Work out the finished part from the listing and answer in its coordinate system (mm). A direction names the side the tool comes from. Give positions to 0.01 mm unless a question says otherwise; leave off trailing zeros. Loops run counter-clockwise (first coordinate to the right, second up) from the corner with the lowest first, then second, coordinate; pieces in that order, holes last. Notation, with made-up numbers: (50, 39.25) - (85, 39.25) arc R18 ccw to (85, 66.25) - close; hole circle Ø4 at (-32.5, 72.5). An arc over 180 degrees is marked (long way). One line per item, written item: value.
from build123d import *

# Parameters (mm, degrees)
SKETCH1_W           = 182.88
SKETCH1_H           = 76.2
BOSS_EXTRUDE1_DEPTH = 10
SKETCH2_W           = 40
SKETCH2_H           = 12.7
BOSS_EXTRUDE2_DEPTH = 129.7
SKETCH3_W           = 80.079962719
SKETCH3_H           = 42.379632712
BOSS_EXTRUDE3_DEPTH = 12.7
SKETCH4_W           = 38.600527556
SKETCH4_H           = 39.516860555
BOSS_EXTRUDE4_DEPTH = 12.7
SKETCH6_W           = 45.336351273
SKETCH6_H           = 46.321924127
BOSS_EXTRUDE5_DEPTH = 63.5
SKETCH7_R           = 6.35
BOSS_EXTRUDE6_DEPTH = 99.06


with BuildPart() as part:
    # Sketch1 → Boss-Extrude1 (new body)
    with BuildSketch(Plane(origin=(0, 0, 0), x_dir=(1, 0, 0), z_dir=(0, 1, 0))):
        with Locations((91.44, 38.1)):
            Rectangle(SKETCH1_W, SKETCH1_H)
    extrude(amount=BOSS_EXTRUDE1_DEPTH)

    # Sketch2 → Boss-Extrude2 (add)
    with BuildSketch(Plane(origin=(0, 10, 0), x_dir=(1, 0, 0), z_dir=(0, 1, 0))):
        with Locations((135.159453347, 69.85)):
            Rectangle(SKETCH2_W, SKETCH2_H)
    extrude(amount=BOSS_EXTRUDE2_DEPTH)

    # Sketch3 → Boss-Extrude3 (add)
    with BuildSketch(Plane(origin=(0, 0, -76.2), x_dir=(-1, 0, 0), z_dir=(0, 0, -1))):
        with Locations((-115.119471988, 112.229632712)):
            Rectangle(SKETCH3_W, SKETCH3_H)
    extrude(amount=-BOSS_EXTRUDE3_DEPTH)

    # Sketch4 → Boss-Extrude4 (add)
    with BuildSketch(Plane.XY.offset(-63.5)):
        with Locations((95.110147759, 112.061245717)):
            Rectangle(SKETCH4_W, SKETCH4_H)
    extrude(amount=BOSS_EXTRUDE4_DEPTH)

    # Sketch6 → Boss-Extrude5 (add)
    with BuildSketch(Plane.XY.offset(-50.8)):
        with Locations((94.988062274, 111.441174429)):
            Rectangle(SKETCH6_W, SKETCH6_H)
    extrude(amount=BOSS_EXTRUDE5_DEPTH)

    # Sketch7 → Boss-Extrude6 (add)
    with BuildSketch(Plane.XY.offset(12.7)):
        with Locations((94.988062274, 111.441174429)):
            Circle(SKETCH7_R)
    extrude(amount=-BOSS_EXTRUDE6_DEPTH)


solid = part.part
1. The mould has two halves that part along Y. Classify faces 6 (the flat face through (135, 139.7, -70)), 7 (the flat face through (95, 92.303, -57)), 8 (the flat face through (95, 88.28, -19)), 9 (the flat face through (117.656, 111, -19)): released by +Y, released by -Y, zero draft, split by the parting line, or undercut.
Output:
face 6: released by +Y
face 7: undercut
face 8: undercut
face 9: zero draft
2. Find the intervals of material crossed by line 1 along Y through (x, z) = (117, -9); line 2 along Z through (x, y) = (85.5, 92); line 3 along Y through (x, z) = (83, -61.5), in increasing order.
Output:
line 1: y = 0 to 10, 88.28 to 134.6
line 2: z = -76.2 to -63.5, -50.8 to 12.7
line 3: y = 0 to 10, 92.3 to 131.82
3. Section C-C (y = 96) is taken. Write down the section's boundary in (x, z).
Output:
outline: (72.32, -50.8) - (75.81, -50.8) - (75.81, -63.5) - (75.08, -63.5) - (75.08, -76.2) - (155.16, -76.2) - (155.16, -63.5) - (114.41, -63.5) - (114.41, -50.8) - (117.66, -50.8) - (117.66, 12.7) - (72.32, 12.7) - close
4. Section D-D (z = -67.5) is taken. Write down the section's boundary in (x, y), and give its area (3 significant figures).
Output:
outline: (0, 0) - (182.88, 0) - (182.88, 10) - (155.16, 10) - (155.16, 139.7) - (115.16, 139.7) - (115.16, 133.42) - (75.08, 133.42) - (75.08, 91.04) - (115.16, 91.04) - (115.16, 10) - (0, 10) - close
area: 8,720 mm²
5. Section B-B (x = 86) is taken. Write down the section's boundary in (y, z).
Output:
outline: (0, -76.2) - (10, -76.2) - (10, 0) - (0, 0) - close; (88.28, -50.8) - (92.3, -50.8) - (92.3, -63.5) - (91.04, -63.5) - (91.04, -76.2) - (133.42, -76.2) - (133.42, -63.5) - (131.82, -63.5) - (131.82, -50.8) - (134.6, -50.8) - (134.6, 12.7) - (88.28, 12.7) - close
6. Section A-A (z = -39) is taken. Write down the section's boundary in (x, y), and give its area (3 significant figures).
Output:
outline: (0, 0) - (182.88, 0) - (182.88, 10) - (0, 10) - close; (72.32, 88.28) - (117.66, 88.28) - (117.66, 134.6) - (72.32, 134.6) - close
area: 3,930 mm²
7. For faces 1 (the cylindrical face through (93.612, 105.242, -81.209)), 2 (the flat face through (75.81, 112, -57)), 3 (the flat face through (115.159, 137, -70)), 4 (the flat face through (114.41, 112, -57)), 5 (the flat face through (155.159, 74, -70)), determine the directions among +Z, -Z, +X, -X, +Y, -Y from which every point of the face is accessible in a straight line to the end or side of a thin tool.
Output:
face 1: -Z
face 2: -X, +Y
face 3: -Z, -X, +Y
face 4: +X, +Y
face 5: +Z, -Z, +X, +Y
8. Flat-ended cylindrical pins translate along their axes: pin 1 Ø1 at (x, z) = (53.5, -59.5) entering from +Y; pin 2 Ø23 at (y, z) = (102.5, -32.5) entering from -X; pin 3 Ø6.5 at (x, z) = (92.5, -69.5) entering from -Y; pin 4 Ø10 at (y, z) = (114, -72.5) entering from -X. Find the tip coordinate at first contact, or state that the pin passes through.
Output:
pin 1: stops at y = 10
pin 2: stops at x = 72.32
pin 3: stops at y = 0
pin 4: stops at x = 75.08
